Geometry: final body of the model. Coordinates: model frame, mm. Face numbers are marked on the shaded views. A direction names the side the tool comes from. Coordinates: 2 decimals unless noted, no trailing zeros. Loops run counter-clockwise (first coordinate to the right, second up) from the corner with the lowest first, then second, coordinate; pieces in that order, holes last. Notation, with made-up numbers: (37.5, 50) - (46.5, 50) arc R20 ccw to (46.5, 83) - close; hole circle Ø1 at (-32, -13.5). An arc over 180 degrees is marked (long way). Answer in a Markdown table with one row per item.
from build123d import *

# Parameters (mm, degrees)
SKETCH1_R           = 30
SKETCH1_R_2         = 10
BOSS_EXTRUDE1_DEPTH = 12.5
SKETCH2_R           = 22.5
CUT_EXTRUDE1_DEPTH  = 10
SKETCH3_R           = 2.5
CUT_EXTRUDE2_DEPTH  = 16
CIRPATTERN3_COUNT   = 5
CIRPATTERN2_COUNT   = 5


with BuildPart() as part:
    # Sketch1 → Boss-Extrude1 (new body, symmetric)
    with BuildSketch(Plane.XY):
        Circle(SKETCH1_R)
        Circle(SKETCH1_R_2, mode=Mode.SUBTRACT)
    extrude(amount=BOSS_EXTRUDE1_DEPTH, both=True)

    # Sketch2 → Cut-Extrude1 (cut)
    with BuildSketch(Plane(origin=(0, 0, -12.5), x_dir=(-1, 0, 0), z_dir=(0, 0, -1))):
        Circle(SKETCH2_R)
    cut_extrude1 = extrude(amount=-CUT_EXTRUDE1_DEPTH, mode=Mode.SUBTRACT)

    # Mirror1: Cut-Extrude1 across plane
    add(cut_extrude1.mirror(Plane.XY), mode=Mode.SUBTRACT)

    # Sketch3 → Cut-Extrude2 (cut, through all)
    with BuildSketch(Plane(origin=(0, 0, -2.5), x_dir=(-1, 0, 0), z_dir=(0, 0, -1))):
        with Locations((0, 15)):
            Circle(SKETCH3_R)
    cut_extrude2 = extrude(amount=-CUT_EXTRUDE2_DEPTH, mode=Mode.SUBTRACT)

    # CirPattern3: Cut-Extrude2 ×5 about axis
    cirpattern3_axis = Axis((0, 0, 0), (0, 0, 1))
    for i in range(1, CIRPATTERN3_COUNT):
        add(cut_extrude2.rotate(cirpattern3_axis, i * 360 / CIRPATTERN3_COUNT), mode=Mode.SUBTRACT)

    # CirPattern2: part ×5 about axis
    cirpattern2_axis = Axis((0, 0, 0), (0, 0, 1))


with BuildPart() as part_1:
    add(part.part)
    for i in range(1, CIRPATTERN2_COUNT):
        add(part.part.rotate(cirpattern2_axis, i * 360 / CIRPATTERN2_COUNT))


solid = part_1.part
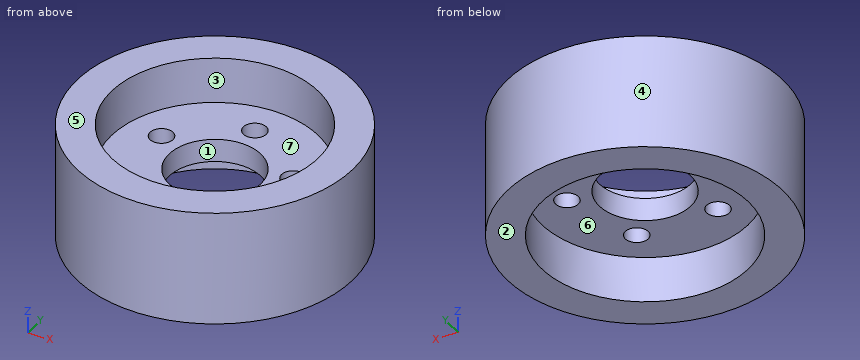
(1) Cut plane A-A on x = 0. Output: boundary loops of the cut face in (y, z).
Verdict:
| item | result |
|---|---|
| outline | (-30, -12.5) - (-22.5, -12.5) - (-22.5, -2.5) - (-10, -2.5) - (-10, 2.5) - (-22.5, 2.5) - (-22.5, 12.5) - (-30, 12.5) - close; (10, -2.5) - (12.5, -2.5) - (12.5, 2.5) - (10, 2.5) - close; (17.5, -2.5) - (22.5, -2.5) - (22.5, -12.5) - (30, -12.5) - (30, 12.5) - (22.5, 12.5) - (22.5, 2.5) - (17.5, 2.5) - close |
(2) First-contact query: pin 1 Ø4 at (x, z) = (20, -7) entering from +Y; pin 2 Ø6.5 at (x, y) = (0, 15) entering from +Z; pin 3 Ø4.5 at (x, y) = (-14.27, 4.64) entering from +Z; pin 4 Ø1.5 at (x, z) = (4.5, 6) entering from +Y. Flat tips, straight axial feed; report the tip coordinate or a pass-through.
Verdict:
| item | result |
|---|---|
| pin 1 | stops at y = 24 |
| pin 2 | stops at z = 2.5 |
| pin 3 | passes through |
| pin 4 | stops at y = 29.76 |
(3) Ray query, probe 1 along Y at (x, z) = (0, 0.85); probe 2 along X at (y, z) = (0, -7.5); probe 3 along Y at (x, z) = (7.5, -0.75). Return the intervals inside material, ascending.
Verdict:
| item | result |
|---|---|
| probe 1 | y = -30 to -10, 10 to 12.5, 17.5 to 30 |
| probe 2 | x = -30 to -22.5, 22.5 to 30 |
| probe 3 | y = -29.05 to -14.26, -10.01 to -6.61, 6.61 to 29.05 |
(4) Cut plane B-B on y = 0. Output: boundary loops of the cut face in (x, z), then the cut area to 3 significant figures.
Verdict:
| item | result |
|---|---|
| outline | (-30, -12.5) - (-22.5, -12.5) - (-22.5, -2.5) - (-10, -2.5) - (-10, 2.5) - (-22.5, 2.5) - (-22.5, 12.5) - (-30, 12.5) - close; (10, -2.5) - (22.5, -2.5) - (22.5, -12.5) - (30, -12.5) - (30, 12.5) - (22.5, 12.5) - (22.5, 2.5) - (10, 2.5) - close |
| area | 500 mm² |
(5) Access query for the marked faces 5, 6 and 7. Directions: +Z, -Z, +X, -X, +Y, -Y. A direction counts if a zero-diameter tool reaches every point of the face in a straight line with its end or side. Return the directions, or none.
Verdict:
| item | result |
|---|---|
| face 5 | +Z, +X, -X, +Y, -Y |
| face 6 | -Z |
| face 7 | +Z |
(6) Cut plane D-D on z = -3.5. Output: boundary loops of the cut face in (x, y), then the cut area to 3 significant figures.
Verdict:
| item | result |
|---|---|
| outline | circle Ø60 at (0, 0); hole circle Ø45 at (0, 0) |
| area | 1,240 mm² |
(7) Pull-direction query (Y, two-part tool) for the marked faces 1, 2, 3 and 4; classes: pulls with the +Y half, pulls with the -Y half, needs draft (parallel to the pull), parting line crosses it, or undercut.
Verdict:
| item | result |
|---|---|
| face 1 | undercut |
| face 2 | needs draft |
| face 3 | undercut |
| face 4 | parting line crosses it |
(8) Cut plane C-C on z = 0.5. Output: boundary loops of the cut face in (x, y), then the cut area to 3 significant figures.
Verdict:
| item | result |
|---|---|
| outline | circle Ø60 at (0, 0); hole circle Ø5 at (-14.27, 4.64); hole circle Ø5 at (-8.82, -12.14); hole circle Ø20 at (0, 0); hole circle Ø5 at (0, 15); hole circle Ø5 at (8.82, -12.14); hole circle Ø5 at (14.27, 4.64) |
| area | 2,420 mm² |
